```python
from build123d import *

# Parameters (mm, degrees)
RESSALTO_EXTRUS_O1_DEPTH = 10
ESBO_O2_W                = 5
ESBO_O2_H                = 21.6
RESSALTO_EXTRUS_O2_DEPTH = 50.4


with BuildPart() as part:
    # Esboço1 → Ressalto-extrusão1 (new body)
    with BuildSketch(Plane(origin=(0, 0, 0), x_dir=(1, 0, 0), z_dir=(0, 1, 0))):
        Polygon((-10.8, 22.3), (-10.8, 10.8), (-22.3, 10.8), (-22.3, -10.8), (-10.8, -10.8), (-10.8, -22.3), (10.8, -22.3), (10.8, -10.8), (22.3, -10.8), (22.3, 10.8), (10.8, 10.8), (10.8, 22.3), align=None)
    extrude(amount=RESSALTO_EXTRUS_O1_DEPTH)

    # Esboço2 → Ressalto-extrusão2 (add)
    with BuildSketch(Plane(origin=(0, 0, 0), x_dir=(1, 0, 0), z_dir=(0, 1, 0))):
        with Locations((24.8, 0)):
            Rectangle(ESBO_O2_W, ESBO_O2_H)
        with Locations((-24.8, 0)):
            Rectangle(ESBO_O2_W, ESBO_O2_H)
    extrude(amount=RESSALTO_EXTRUS_O2_DEPTH)


solid = part.part
```
Could you check a few things on this model? Use its own coordinates, in mm. A direction names the side the tool comes from. Give positions to 0.01 mm unless a question says otherwise; leave off trailing zeros. Loops run counter-clockwise (first coordinate to the right, second up) from the corner with the lowest first, then second, coordinate; pieces in that order, holes last. Notation, with made-up numbers: (71.5, 36) - (95.5, 36) arc R22 cw to (95.5, 52) - close; hole circle Ø6 at (43.25, 67). An arc over 180 degrees is marked (long way). Answer in a Markdown table with one row per item. Add a question column.
Q1. If we section it at C-C (y = 5.5): List the corners of the cut face in (x, z) for me, plus the area to 3 significant figures.
Q2. For pin 1 (3 mm diameter, centred on y = 4.5, z = 16, fed in from +X); pin 2 (8 mm diameter, centred on x = -20, y = 19, fed in from +Z); pin 3 (2 mm diameter, centred on x = -8, z = -16, fed in from -Y); pin 4 (11 mm diameter, centred on y = 3, z = 18.5, fed in from -X), each with a flat end and sliding along its axis, tell me the tip position at first contact or that it passes through.
Q3. If we section it at D-D (x = 0): List the corners of the cut face in (y, z) for me, plus the area to 3 significant figures.
Q4. Which directions (+Z, -Z, +X, -X, +Y, -Y) give clear straight access to the entire face, cutting with the end or side of a thin tool? Please do faces 1 (the face through (0, 10, 0)), 2 (the face through (23, 19, -10.8)), 3 (the face through (-23, 19, 10.8)), 4 (the face through (23, 19, 10.8)).
Q5. If we section it at B-B (z = 10): List the corners of the cut face in (x, y) for me, plus the area to 3 significant figures.
Q6. We'd pull the mould along X, two halves only. Please class faces 5 (the face through (-10.8, 5, 16)), 6 (the face through (-23, 19, -10.8)), 7 (the face through (-22.3, 30, 0)), 8 (the face through (22.3, 30, 0)): +X half, -X half, draft (parallel to the pull), parting line (faces both ways), or undercut.
Q7. Please list where these lines run through material, in increasing order: L1, parallel to X at y = 33.5, z = -1.5; L2, parallel to Y at x = -19, z = -10; L3, parallel to Z at x = 14, y = 9. Write a range as from..to.
Q8. If we section it at A-A (y = 22): List the corners of the cut face in (x, z) for me.
The answers:
| question | item | result |
|---|---|---|
| 1 | outline | (-27.3, -10.8) - (-10.8, -10.8) - (-10.8, -22.3) - (10.8, -22.3) - (10.8, -10.8) - (27.3, -10.8) - (27.3, 10.8) - (10.8, 10.8) - (10.8, 22.3) - (-10.8, 22.3) - (-10.8, 10.8) - (-27.3, 10.8) - close |
| 1 | area | 1,680 mm^2 |
| 2 | pin 1 | stops at x = 10.8 |
| 2 | pin 2 | stops at z = 10.8 |
| 2 | pin 3 | stops at y = 0 |
| 2 | pin 4 | stops at x = -10.8 |
| 3 | outline | (0, -22.3) - (10, -22.3) - (10, 22.3) - (0, 22.3) - close |
| 3 | area | 446 mm^2 |
| 4 | face 1 | +Z, -Z, +Y |
| 4 | face 2 | -Z, +X, +Y, -Y |
| 4 | face 3 | +Z, -X, +Y, -Y |
| 4 | face 4 | +Z, +X, +Y, -Y |
| 5 | outline | (-27.3, 0) - (27.3, 0) - (27.3, 50.4) - (22.3, 50.4) - (22.3, 10) - (-22.3, 10) - (-22.3, 50.4) - (-27.3, 50.4) - close |
| 5 | area | 950 mm^2 |
| 6 | face 5 | -X half |
| 6 | face 6 | draft |
| 6 | face 7 | undercut |
| 6 | face 8 | undercut |
| 7 | L1 | x = -27.3..-22.3, 22.3..27.3 |
| 7 | L2 | y = 0..10 |
| 7 | L3 | z = -10.8..10.8 |
| 8 | outline | (-27.3, -10.8) - (-22.3, -10.8) - (-22.3, 10.8) - (-27.3, 10.8) - close; (22.3, -10.8) - (27.3, -10.8) - (27.3, 10.8) - (22.3, 10.8) - close |
